Source: three-view drawing plus pictorial views. Frame: mm from the lowest corner of the part. A direction names the side the tool comes from. Round coordinates to 2 decimals unless told otherwise and drop trailing zeros. Loops run counter-clockwise (first coordinate to the right, second up) from the corner with the lowest first, then second, coordinate; pieces in that order, holes last. Notation, with made-up numbers: (58.5, 11) -> (91.5, 11) arc R34 ccw to (91.5, 50) -> close; hole circle Ø9 at (-35.5, -33.5). An arc over 180 degrees is marked (long way). Answer in a Markdown table with one row per item.
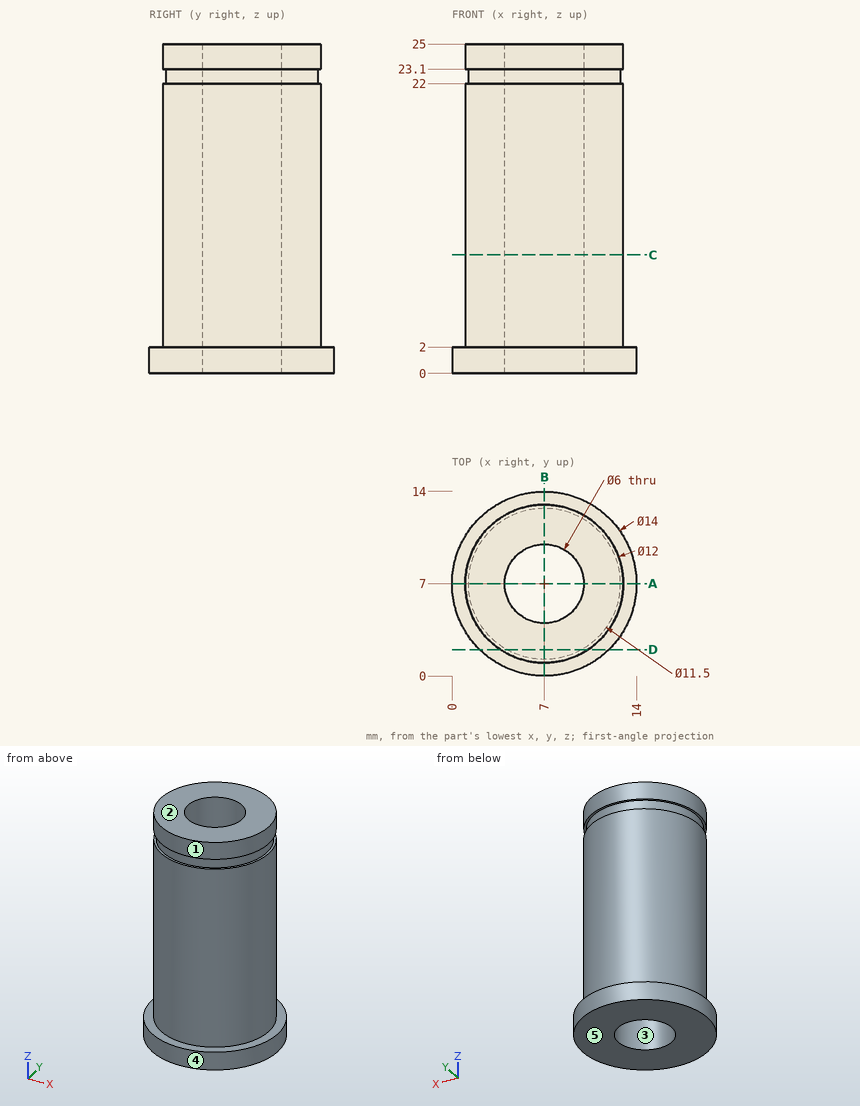
Item 1: Line query: probe 1 along Y at (x, z) = (7, 12); probe 2 along X at (y, z) = (6.5, 8); probe 3 along Y at (x, z) = (5.75, 9). Output: solid intervals per line, ascending. Write a range as [from, to].
Answer:
| item | result |
|---|---|
| probe 1 | y = [1, 4], [10, 13] |
| probe 2 | x = [1.02, 4.04], [9.96, 12.98] |
| probe 3 | y = [1.13, 4.27], [9.73, 12.87] |
Item 2: Cut plane A-A (y = 7). Output: boundary loops of the cut face in (x, z).
Answer:
| item | result |
|---|---|
| outline | (0, 0) -> (4, 0) -> (4, 25) -> (1, 25) -> (1, 23.1) -> (1.25, 23.1) -> (1.25, 22) -> (1, 22) -> (1, 2) -> (0, 2) -> close; (10, 0) -> (14, 0) -> (14, 2) -> (13, 2) -> (13, 22) -> (12.75, 22) -> (12.75, 23.1) -> (13, 23.1) -> (13, 25) -> (10, 25) -> close |
Item 3: Reachability of the marked faces 1 and 2 from +Z, -Z, +X, -X, +Y, -Y: full face, straight path, thin tool, end or side. Return the list, or none.
Answer:
| item | result |
|---|---|
| face 1 | +Z |
| face 2 | +Z, +X, -X, +Y, -Y |
Item 4: Pin query (flat end, axial travel): pin 1 Ø7 at (x, y) = (7, 7.5) entering from +Z; pin 2 Ø1 at (x, z) = (2, 15.5) entering from +Y; pin 3 Ø8 at (x, z) = (3.5, 6.5) entering from -Y; pin 4 Ø4 at (x, z) = (10, 12) entering from -Y. Return the tip coordinate at first contact, or that it passes through.
Answer:
| item | result |
|---|---|
| pin 1 | stops at z = 25 |
| pin 2 | stops at y = 10.97 |
| pin 3 | stops at y = 1 |
| pin 4 | stops at y = 1.08 |
Item 5: Draft query along X for the marked faces 3, 4 and 5. Return one class per face: pulls with the +X half, pulls with the -X half, needs draft (parallel to the pull), parting line crosses it, or undercut.
Answer:
| item | result |
|---|---|
| face 3 | undercut |
| face 4 | parting line crosses it |
| face 5 | needs draft |
Item 6: Cut plane C-C (z = 9). Output: boundary loops of the cut face in (x, y), then the cut area to 3 significant figures.
Answer:
| item | result |
|---|---|
| outline | circle Ø12 at (7, 7); hole circle Ø6 at (7, 7) |
| area | 84.8 mm² |
Item 7: Cut plane D-D (y = 2). Output: boundary loops of the cut face in (x, z).
Answer:
| item | result |
|---|---|
| outline | (2.1, 0) -> (11.9, 0) -> (11.9, 2) -> (10.32, 2) -> (10.32, 22) -> (9.84, 22) -> (9.84, 23.1) -> (10.32, 23.1) -> (10.32, 25) -> (3.68, 25) -> (3.68, 23.1) -> (4.16, 23.1) -> (4.16, 22) -> (3.68, 22) -> (3.68, 2) -> (2.1, 2) -> close |
